Verification items for the finished model (mm, model axes). A direction names the side the tool comes from. Round coordinates to 2 decimals unless told otherwise and drop trailing zeros. Order: outer loops, then holes, each group sorted by start corner. A loop starts at its lowest first (then second) coordinate and runs counter-clockwise, first axis right, second up. Notation, with made-up numbers: (-13.5, 83) -> (-7.5, 83) arc R7 ccw to (-7.5, 94) -> close; hole circle Ø2 at (69.25, 22.25). An arc over 180 degrees is marked (long way). Put each result on its own line as item: value.
from build123d import *

# Parameters (mm, degrees)
SKETCH_1_W          = 200
SKETCH_1_H          = 180
EXTRUDE_1_DEPTH     = 5
SKETCH_2_R          = 2
CUT_EXTRUDE_1_DEPTH = 135.629120178
FILLET_1_R          = 10
SKETCH_3_W          = 30
SKETCH_3_H          = 115
CUT_EXTRUDE_2_DEPTH = 135.629120178
CUT_EXTRUDE_3_DEPTH = 135.629120178
FILLET_2_R          = 8
FILLET_3_R          = 15


with BuildPart() as part:
    # Sketch 1 → Extrude 1 (new body)
    with BuildSketch(Plane.XY):
        Rectangle(SKETCH_1_W, SKETCH_1_H)
    extrude(amount=EXTRUDE_1_DEPTH)

    # Sketch 2 → Cut-Extrude 1 (cut, through all)
    with BuildSketch(Plane.XY.offset(5)):
        with Locations((-70, 84)):
            Circle(SKETCH_2_R)
        with Locations((-70, 72)):
            Circle(SKETCH_2_R)
        with Locations((-55, 84)):
            Circle(SKETCH_2_R)
        with Locations((-55, 72)):
            Circle(SKETCH_2_R)
        with Locations((-5, 84)):
            Circle(SKETCH_2_R)
        with Locations((-5, 72)):
            Circle(SKETCH_2_R)
        with Locations((55, 84)):
            Circle(SKETCH_2_R)
        with Locations((55, 72)):
            Circle(SKETCH_2_R)
    extrude(amount=-CUT_EXTRUDE_1_DEPTH, mode=Mode.SUBTRACT)

    # Fillet 1
    fillet_1_edges = [part.edges().sort_by_distance(p)[0] for p in [
        (-100, 90, 2.5),
        (100, 90, 2.5),
        (100, -90, 2.5),
        (-100, -90, 2.5),
    ]]
    fillet(fillet_1_edges, radius=FILLET_1_R)

    # Sketch 3 → Cut-Extrude 2 (cut, through all)
    with BuildSketch(Plane.XY.offset(5)):
        with Locations((85, -32.5)):
            Rectangle(SKETCH_3_W, SKETCH_3_H)
    extrude(amount=-CUT_EXTRUDE_2_DEPTH, mode=Mode.SUBTRACT)

    # Sketch 4 → Cut-Extrude 3 (cut, through all)
    with BuildSketch(Plane.XY.offset(5)):
        Polygon((70, 25), (5, -90), (70, -90), align=None)
    extrude(amount=-CUT_EXTRUDE_3_DEPTH, mode=Mode.SUBTRACT)

    # Fillet 2
    fillet_2_edges = [part.edges().sort_by_distance(p)[0] for p in [
        (100, 25, 2.5),
        (70, 25, 2.5),
    ]]
    fillet(fillet_2_edges, radius=FILLET_2_R)

    # Fillet 3
    fillet_3_edges = [part.edges().sort_by_distance(p)[0] for p in [
        (5, -90, 2.5),
    ]]
    fillet(fillet_3_edges, radius=FILLET_3_R)


solid = part.part
Item 1: Material ranges on L1, parallel to Y at x = -55, z = 1.05; L2, parallel to Y at x = 55, z = 4; L3, parallel to Y at x = 7, z = 4.45, recorded low to high. Write a range as [from, to].
Check sheet entries:
L1: y = [-90, 70], [74, 82], [86, 90]
L2: y = [-1.54, 70], [74, 82], [86, 90]
L3: y = [-85.46, 90]
Item 2: Section check C-C on x = 25. Record the boundary of the cut face in (y, z), then the cut area to 3 significant figures.
Check sheet entries:
outline: (-54.62, 0) -> (90, 0) -> (90, 5) -> (-54.62, 5) -> close
area: 723 mm^2
Item 3: Tool access check on faces 1 (the flat face through (83, 25, 3)), 2 (the flat face through (-100, -1, 2)). Record the directions out of +Z, -Z, +X, -X, +Y, -Y that give a thin tool (end or side, any length) a straight path to the whole face; none if there is none.
Check sheet entries:
face 1: +Z, -Z, +X, -Y
face 2: +Z, -Z, -X, +Y, -Y
Item 4: Section check B-B on y = 17.5. Record the boundary of the cut face in (x, z), then the cut area to 3 significant figures.
Check sheet entries:
outline: (-100, 0) -> (65.76, 0) -> (65.76, 5) -> (-100, 5) -> close
area: 829 mm^2
Item 5: Section check A-A on z = 3.55. State how many separate pieces and enclosed holes the cut face has, then the cut area to 3 significant figures.
Check sheet entries:
separate pieces: 1
enclosed holes: 8
area: 28,600 mm^2
Item 6: Gauge pin test, flat ends, axial feed: pin 1 Ø10 at (x, y) = (-2, 41.5) entering from -Z; pin 2 Ø2.5 at (x, y) = (-55, 72) entering from -Z. Record the tip position at first contact, or that the pin passes through.
Check sheet entries:
pin 1: stops at z = 0
pin 2: passes through
